```python
from build123d import *

# Parameters (mm, degrees)
SKETCH1_R            = 60
SKETCH1_R_2          = 7.9
BOSS_EXTRUDE1_DEPTH  = 8
SKETCH2_R            = 1.7
CUT_EXTRUDE1_DEPTH   = 9
SKETCH3_R            = 3.4
CUT_EXTRUDE2_DEPTH   = 3
M6_CLEARANCE_HOLE1_D = 6.6


with BuildPart() as part:
    # Sketch1 → Boss-Extrude1 (new body)
    with BuildSketch(Plane.XY):
        Circle(SKETCH1_R)
        Circle(SKETCH1_R_2, mode=Mode.SUBTRACT)
    extrude(amount=BOSS_EXTRUDE1_DEPTH)

    # Sketch2 → Cut-Extrude1 (cut, through all)
    with BuildSketch(Plane.XY.offset(8)):
        with Locations((0, 12.5)):
            Circle(SKETCH2_R)
        with Locations((0, -12.5)):
            Circle(SKETCH2_R)
    extrude(amount=-CUT_EXTRUDE1_DEPTH, mode=Mode.SUBTRACT)

    # Sketch3 → Cut-Extrude2 (cut)
    with BuildSketch(Plane.XY.offset(8)):
        with Locations((29.781294677, -3.615866061)):
            Circle(SKETCH3_R)
        with Locations((24.689650078, -17.041748121)):
            Circle(SKETCH3_R)
        with Locations((13.941904189, -26.563571062)):
            Circle(SKETCH3_R)
        with Locations((0.000236068, -29.999999999)):
            Circle(SKETCH3_R)
        with Locations((-13.941486133, -26.563790475)):
            Circle(SKETCH3_R)
        with Locations((-24.689381874, -17.042136682)):
            Circle(SKETCH3_R)
        with Locations((-29.781237767, -3.616334754)):
            Circle(SKETCH3_R)
        with Locations((-28.050570991, 10.637925883)):
            Circle(SKETCH3_R)
        with Locations((-19.893856446, 22.455165902)):
            Circle(SKETCH3_R)
        with Locations((-7.179699137, 29.128198027)):
            Circle(SKETCH3_R)
        with Locations((7.17924072, 29.128311017)):
            Circle(SKETCH3_R)
        with Locations((19.893503047, 22.455478987)):
            Circle(SKETCH3_R)
        with Locations((28.050403569, 10.638367338)):
            Circle(SKETCH3_R)
    extrude(amount=-CUT_EXTRUDE2_DEPTH, mode=Mode.SUBTRACT)

    # M6 Clearance Hole1 (through all)
    with Locations(Plane.XY.offset(8)):
        with Locations((-37.123106012, 37.123106012), (0, 52.5), (37.123106012, 37.123106012), (52.5, 0), (37.123106012, -37.123106012), (0, -52.5), (-37.123106012, -37.123106012), (-52.5, 0)):
            Hole(M6_CLEARANCE_HOLE1_D / 2)


solid = part.part
```
CAD build for the part. Positions are in the model's coordinates, mm. A direction names the side the tool comes from. Give positions to 0.01 mm unless a question says otherwise; leave off trailing zeros. Order: outer loops, then holes, each group sorted by start corner. A loop starts at its lowest first (then second) coordinate and runs counter-clockwise, first axis right, second up.
(1) Tool access for faces 4 (the cylindrical face through (0.43, -49.23, 3.94)), 5 (the cylindrical face through (16.497, 22.605, 6.521)): list every direction of +Z, -Z, +X, -X, +Y, -Y with a clear straight run to the whole face (end or side of a thin tool).
(2) Saw through at B-B, the plane y = -52.5. Give the cut face in (x, z), then the cut area to 3 significant figures.
(3) Saw through at A-A, the plane x = 0. Give the cut face in (y, z).
(4) Flat gauge pins, fed straight in: pin 1 (2 mm diameter, centred on x = 9, y = 30, fed in from +Z); pin 2 (4 mm diameter, centred on y = 30.5, z = 1.5, fed in from -X); pin 3 (1 mm diameter, centred on y = 21, z = 4.5, fed in from -X); pin 4 (4 mm diameter, centred on x = -52.5, y = 0, fed in from -Z). Where does each tip first touch, or does it go through?
(5) Mould opens along X. For faces 1 (the cylindrical face through (-59.94, 2.64, 3.94)), 2 (the flat face through (12, 1, 0)), 3 (the flat face through (-20, 23, 5)) say: released by +X, released by -X, zero draft, split by the parting line, or undercut.
(6) Drill centre lines: L1, parallel to Y at x = 0, z = 2; L2, parallel to Y at x = -37, z = 2.25. Where is each one in solid material? Low to high.
(7) Saw through at D-D, the plane z = 1.5. State how many separate pieces and enclosed holes the cut face has, then the cut area to 3 significant figures.
Results found:
1. face 4: +Z, -Z
1. face 5: +Z
2. outline: (-29.05, 0) - (-3.3, 0) - (-3.3, 8) - (-29.05, 8) - close; (3.3, 0) - (29.05, 0) - (29.05, 8) - (3.3, 8) - close
2. area: 412 mm2
3. outline: (-60, 0) - (-55.8, 0) - (-55.8, 8) - (-60, 8) - close; (-49.2, 0) - (-14.2, 0) - (-14.2, 8) - (-26.6, 8) - (-26.6, 5) - (-33.4, 5) - (-33.4, 8) - (-49.2, 8) - close; (-10.8, 0) - (-7.9, 0) - (-7.9, 8) - (-10.8, 8) - close; (7.9, 0) - (10.8, 0) - (10.8, 8) - (7.9, 8) - close; (14.2, 0) - (49.2, 0) - (49.2, 8) - (14.2, 8) - close; (55.8, 0) - (60, 0) - (60, 8) - (55.8, 8) - close
4. pin 1: stops at z = 5
4. pin 2: stops at x = -52.8
4. pin 3: stops at x = -56.39
4. pin 4: passes through
5. face 1: split by the parting line
5. face 2: zero draft
5. face 3: undercut
6. L1: y = -60 to -55.8, -49.2 to -14.2, -10.8 to -7.9, 7.9 to 10.8, 14.2 to 49.2, 55.8 to 60
6. L2: y = -47.23 to -40.42, -33.83 to 33.83, 40.42 to 47.23
7. separate pieces: 1
7. enclosed holes: 11
7. area: 10,800 mm2
